Autodesk Inventor part; units mm, degrees
ref_plane "Work Plane1" through (29, 0, 0) normal (0, -1, 0) x (1, 0, 0)
ref_plane "YZ Plane" through (0, 0, 0) normal (1, 0, 0) x (0, 1, 0)
ref_plane "XZ Plane" through (0, 0, 0) normal (0, 1, 0) x (-1, 0, 0)
sketch "Sketch1" plane through (0, 0, 0) normal (0, 0, 1) x (1, 0, 0)
  line L0 (-1.1667, 0) -> (30, 0)
  line L1 (30, 0) -> (30, 2.5)
  line L2 (30, 2.5) -> (14, 2.5)
  line L3 (14, 2.5) -> (13.5091, 2.5)
  line L4 (13.5091, 2.5) -> (0, 2.5)
  line L5 (0, 2.5) -> (0, 4.25)
  line L6 (0, 4.25) -> (-5, 4.25)
  line L7 (-5, 4.25) -> (-5, 2.3094)
  line L8 (-5, 2.3094) -> (-2.5, 2.3094)
  line L9 (-2.5, 2.3094) -> (-1.1667, 0)
  line L10 (-12, 0) -> (37, 0)
  line L11 (0, -0.85) -> (0, 5.1)
  line L12 (14, 2.5) -> (0, 2.5) construction
  dimension "d1" = 16
  dimension "d2" = 0.4909
  dimension "d3" = 5
  dimension "d4" = 2.5
  dimension "d5" = 60
  dimension "d6" = 5
  dimension "d7" = 5
  dimension "d8" = 4.6188
  dimension "d9" = 8.5
  dimension "d26" = 30
revolve "Body" add sketch "Sketch1" angle 360 about axis through (-1.1667, 0, 0) along (1, 0, 0)
sketch "Sketch2" plane through (-5, 0, 0) normal (-1, 0, 0) x (0, 0, 1)
  circle A0 centre (0, 0) radius 2.3094
  line L0 (0, -5.95) -> (0, 5.95)
  line L1 (-5.95, 0) -> (5.95, 0)
  line L2 (2.3094, 0) -> (1.1547, -2)
  line L3 (1.1547, -2) -> (-1.1547, -2)
  line L4 (-1.1547, -2) -> (-2.3094, 0)
  line L5 (-2.3094, 0) -> (-1.1547, 2)
  line L6 (-1.1547, 2) -> (1.1547, 2)
  line L7 (1.1547, 2) -> (2.3094, 0)
extrude "Slot" add sketch "Sketch2" against normal up to next contours L7 A0 | A0 L2 | L6 L0 A0 | A0 L0 L3 | L0 L6 A0 | A0 L3 L0 | L4 A0 | A0 L5
fillet "Fillet1" radius 0.5 1 edges at (-5, -4.25, 0)
thread "Thread"
chamfer "Chamfer1" distance 0.4908 distance2 0.4908 1 edges at (30, -2.5, 0) measured on face at (30, -0.5525, -0.0341)
ref_plane "Work Plane1" through (29, 0, 0) normal (0, -1, 0) x (1, 0, 0)
fillet "Fillet2" radius 0.1 1 edges at (0, -2.5, 0)
equation "\"d1\" = GEL"
equation "\"d3\" = KOH"
equation "\"d4\" = INTI"
equation "\"d6\" = GD"
equation "\"d7\" = BDM"
equation "\"d8\" = 1.1547 * SW"
equation "\"d9\" = KOD"
equation "\"d26\" = NLG"
equation "\"d30\" = R"
equation "\"d17\" = RR"
equation "\"d13\" = GEL"
equation "\"d15\" = -0.5 * SPD + 0.5 * GD"
equation "\"d16\" = GUL"
equation "\"GD\" = NND"
equation "\"NLG\" = 30"
equation "\"GEL\" = 16"
equation "\"KOD\" = 8.5"
equation "\"KOH\" = NND"
equation "\"INTI\" = 2.5"
equation "\"GAL\" = 0.61345 * PTC"
equation "\"GUL\" = 0.61345 * PTC"
equation "\"BDM\" = NND"
equation "\"SW\" = 4"
equation "\"RR\" = 0.1 * NND"
equation "\"SPD\" = NND - 1.2269 * PTC"
equation "\"R\" = 0.1"
equation "\"PHH\" = 0.13"
equation "\"GD1\" = THREADDIA - 1.2269 * PTC"
equation "\"THREADDIA\" = 5"
equation "\"FAWI\" = 45deg"
equation "\"PTC\" = 0.8"
equation "\"KOH1\" = 4.5"
equation "\"NND\" = 5"
equation "\"TOA\" = 30deg"
equation "\"E0\" = 1.155 * SW"
properties part number "AS 1420 - 1973 - M5 x 30" material "Steel, Mild"
Part model, mm, in its own coordinate system. A direction names the side the tool comes from. Give positions to 0.01 mm unless a question says otherwise; leave off trailing zeros. Write each loop counter-clockwise with the first axis right and the second up, starting at its lowest first coordinate (ties: lowest second). Pieces come first, ordered by that corner, then holes.
1) Probe L1, parallel to X at y = 1.75, z = -3; L2, parallel to Z at x = 10, y = 1.5; L3, parallel to X at y = -0.25, z = 2.25. List the from-to ranges inside material, lowest first.
Resolved:
L1: x = -5 to 0
L2: z = -2 to 2
L3: x = -5 to 29.75
2) Which spindle directions (+Z, -Z, +X, -X, +Y, -Y) get a long thin tool onto all of the face, cutting with end or side? Do faces 4 (the face through (14.6, -0.54, 2.44)), 5 (the face through (30, 0, 0)), 6 (the face through (-4, -2, 0)). Say none if no direction does.
Resolved:
face 4: +X
face 5: +Z, -Z, +X, +Y, -Y
face 6: -X
3) Cut at A-A on x = 5. Write the cut outline in (y, z).
Resolved:
outline: circle Ø5 at (0, 0)
4) Two-plate mould, pull along Y, no slides. Class faces 1 (the face through (-2.282, 2.285, -3.584)), 2 (the face through (0, 2, 2)), 3 (the face through (-3.679, -1.014, -1.724)): released by +Y, released by -Y, zero draft, split by the parting line, or undercut.
Resolved:
face 1: split by the parting line
face 2: zero draft
face 3: undercut
5) Pin check, flat tips, straight feed: pin 1 (2 mm diameter, centred on x = 22, y = 1.5, fed in from -Z); pin 2 (5 mm diameter, centred on x = 19.5, y = -0.5, fed in from +Z); pin 3 (3 mm diameter, centred on x = 12, z = -0.5, fed in from -Y); pin 4 (1.2 mm diameter, centred on x = -4, z = -0.5, fed in from -Y). Stop position of each tip, or through.
Resolved:
pin 1: stops at z = -2.45
pin 2: stops at z = 2.5
pin 3: stops at y = -2.5
pin 4: stops at y = -4.25
